Read the model definition and answer for the solid it produces. Units are mm, in the model's axes. A direction names the side the tool comes from. Round coordinates to 2 decimals unless told otherwise and drop trailing zeros. Write each loop counter-clockwise with the first axis right and the second up, starting at its lowest first coordinate (ties: lowest second). Pieces come first, ordered by that corner, then holes. Notation, with made-up numbers: (32.5, -36.75) -> (39.5, -36.75) arc R24 cw to (39.5, -9.75) -> close; hole circle Ø8 at (35.5, 65.5). An arc over 180 degrees is marked (long way). Return JSON: item names as keys, results as strings.
from build123d import *

# Parameters (mm, degrees)
BOSS_EXTRUDE1_DEPTH = 6.35
SKETCH3_W           = 3.429
SKETCH3_H           = 7.112
CUT_EXTRUDE1_DEPTH  = 20.05
SKETCH4_W           = 7.112
SKETCH4_H           = 3.683
CUT_EXTRUDE2_DEPTH  = 7.35


with BuildPart() as part:
    # Sketch1 → Boss-Extrude1 (new body)
    with BuildSketch(Plane.XY):
        Polygon((0, -19.05), (5.08, -45.466), (13.97, -45.466), (19.05, -19.05), (19.05, 0), (0, 0), align=None)
    extrude(amount=BOSS_EXTRUDE1_DEPTH)

    # Sketch2 → Revolve1 (revolve)
    with BuildSketch(Plane.XY.offset(3.175)):
        with BuildLine():
            Line((9.525, -45.466), (12.7, -45.466))
            Line((12.7, -45.466), (10.588425211, -48.700281514))
            ThreePointArc((10.588425211, -48.700281514), (10.129633144, -49.122834259), (9.525, -49.276))
            Line((9.525, -49.276), (9.525, -45.466))
        make_face()
    revolve(axis=Axis((9.525, -49.276, 3.175), (0, 1, 0)))

    # Sketch3 → Cut-Extrude1 (cut, through all)
    with BuildSketch(Plane.ZY):
        with Locations((3.175, -6.731)):
            Rectangle(SKETCH3_W, SKETCH3_H)
    extrude(amount=-CUT_EXTRUDE1_DEPTH, mode=Mode.SUBTRACT)

    # Sketch4 → Cut-Extrude2 (cut, through all)
    with BuildSketch(Plane.XY.offset(6.35)):
        with Locations((9.525, -17.2085)):
            Rectangle(SKETCH4_W, SKETCH4_H)
    extrude(amount=-CUT_EXTRUDE2_DEPTH, mode=Mode.SUBTRACT)


solid = part.part
Item 1: Section C-C (y = -18) is taken. Give the vertices of the cut face in (x, z).
Worked answers:
{"outline": "(0, 0) -> (5.97, 0) -> (5.97, 6.35) -> (0, 6.35) -> close; (13.08, 0) -> (19.05, 0) -> (19.05, 6.35) -> (13.08, 6.35) -> close"}
Item 2: For a pull along X with two mould halves and no side action, classify faces 4 (the flat face through (9, -7, 4.89)), 5 (the flat face through (9, -15.367, 3)), 6 (the flat face through (0, -12, 3)) as released by +X, released by -X, zero draft, split by the parting line, or undercut.
Worked answers:
{"face 4": "zero draft", "face 5": "undercut", "face 6": "released by -X"}
Item 3: Section A-A (y = -8.5) is taken. Give the vertices of the cut face in (x, z), then the cut area to 3 significant figures.
Worked answers:
{"outline": "(0, 0) -> (19.05, 0) -> (19.05, 1.46) -> (0, 1.46) -> close; (0, 4.89) -> (19.05, 4.89) -> (19.05, 6.35) -> (0, 6.35) -> close", "area": "55.6 mm2"}
Item 4: Straight lines are drawn through the part: L1, parallel to Y at x = 6, z = 3 (3 decimals); L2, parallel to Z at x = 17, y = -4; L3, parallel to Y at x = 9.75, z = 4.25 (3 decimals). For each, find the intervals that lie inside material, in ascending order. Write a range as [from, to].
Worked answers:
{"L1": "y = [-45.466, -19.05], [-15.367, -10.287], [-3.175, 0]", "L2": "z = [0, 1.46], [4.89, 6.35]", "L3": "y = [-48.647, -19.05], [-15.367, -10.287], [-3.175, 0]"}
Item 5: A tool of negligible diameter and unlimited length cuts with its end or side. For faces 1 (the flat face through (13.081, -17, 3)), 2 (the flat face through (10, 0, 3)), 3 (the flat face through (9, -7, 1.46)), from which of +Z, -Z, +X, -X, +Y, -Y can it reach the whole face along a straight path? Write none if from no direction.
Worked answers:
{"face 1": "+Z, -Z", "face 2": "+Z, -Z, +X, -X, +Y", "face 3": "+X, -X"}
Item 6: Flat-ended cylindrical pins translate along their axes: pin 1 (1.3 mm diameter, centred on x = 12.5, z = 3.5, fed in from -Y); pin 2 (1 mm diameter, centred on x = 9.5, z = 2.5, fed in from +Y); pin 3 (3.5 mm diameter, centred on x = 8, z = 2, fed in from -Y). Find the tip coordinate at first contact, or state that the pin passes through.
Worked answers:
{"pin 1": "stops at y = -46.74", "pin 2": "stops at y = 0", "pin 3": "stops at y = -49.26"}
